```python
from build123d import *

# Parameters (mm, degrees)
SKETCH_1_W          = 9
SKETCH_1_H          = 6
EXTRUDE_1_DEPTH     = 1
SKETCH_2_W          = 1
SKETCH_2_H          = 2.206197562
EXTRUDE_2_DEPTH     = 12
CUT_EXTRUDE_1_DEPTH = 0.55
CUT_EXTRUDE_2_DEPTH = 0.55
CUT_EXTRUDE_3_DEPTH = 0.55
CUT_EXTRUDE_START   = -0.55
CUT_EXTRUDE_4_DEPTH = 0.55


with BuildPart() as part:
    # 草圖1 → 填料-伸長1 (new body)
    with BuildSketch(Plane(origin=(0, 0, 0), x_dir=(1, 0, 0), z_dir=(0, 1, 0))):
        Rectangle(SKETCH_1_W, SKETCH_1_H)
    extrude(amount=EXTRUDE_1_DEPTH)

    # 草圖2 → 填料-伸長2 (add)
    with BuildSketch(Plane(origin=(0, 1, 0), x_dir=(1, 0, 0), z_dir=(0, 1, 0))):
        with Locations((-4, 1.896901219)):
            Rectangle(SKETCH_2_W, SKETCH_2_H)
        with Locations((-4, -1.896901219)):
            Rectangle(SKETCH_2_W, SKETCH_2_H)
        with Locations((4, -1.896901219)):
            Rectangle(SKETCH_2_W, SKETCH_2_H)
        with Locations((4, 1.896901219)):
            Rectangle(SKETCH_2_W, SKETCH_2_H)
    extrude(amount=EXTRUDE_2_DEPTH)

    # 草圖4 → 除料-伸長1 (cut)
    with BuildSketch(Plane.XY.offset(-0.793802438)):
        with BuildLine():
            ThreePointArc((4.05, 11.897519797), (3.88890873, 12.286428527), (3.5, 12.447519797))
            Line((3.5, 12.447519797), (3.5, 11.897519797))
            Line((3.5, 11.897519797), (3.5, 11.347519797))
            ThreePointArc((3.5, 11.347519797), (3.88890873, 11.508611068), (4.05, 11.897519797))
        make_face()
        with BuildLine():
            Line((3.5, 11.897519797), (3.5, 12.447519797))
            ThreePointArc((3.5, 12.447519797), (2.95, 11.897519797), (3.5, 11.347519797))
            Line((3.5, 11.347519797), (3.5, 11.897519797))
        make_face()
    extrude(amount=-CUT_EXTRUDE_1_DEPTH, mode=Mode.SUBTRACT)

    # 草圖6 → 除料-伸長2 (cut)
    with BuildSketch(Plane(origin=(0, 0, 0.793802438), x_dir=(-1, 0, 0), z_dir=(0, 0, -1))):
        with BuildLine():
            ThreePointArc((-2.95, 11.9), (-3.11109127, 12.28890873), (-3.5, 12.45))
            Line((-3.5, 12.45), (-3.5, 11.9))
            Line((-3.5, 11.9), (-3.5, 11.35))
            ThreePointArc((-3.5, 11.35), (-3.11109127, 11.51109127), (-2.95, 11.9))
        make_face()
        with BuildLine():
            Line((-3.5, 11.9), (-3.5, 12.45))
            ThreePointArc((-3.5, 12.45), (-4.05, 11.9), (-3.5, 11.35))
            Line((-3.5, 11.35), (-3.5, 11.9))
        make_face()
    extrude(amount=-CUT_EXTRUDE_2_DEPTH, mode=Mode.SUBTRACT)

    # 草圖7 → 除料-伸長3 (cut)
    with BuildSketch(Plane(origin=(0, 0, 0.793802438), x_dir=(-1, 0, 0), z_dir=(0, 0, -1))):
        with BuildLine():
            ThreePointArc((4.05, 11.9), (3.88890873, 12.28890873), (3.5, 12.45))
            Line((3.5, 12.45), (3.5, 11.9))
            Line((3.5, 11.9), (3.5, 11.35))
            ThreePointArc((3.5, 11.35), (3.88890873, 11.51109127), (4.05, 11.9))
        make_face()
        with BuildLine():
            Line((3.5, 11.9), (3.5, 12.45))
            ThreePointArc((3.5, 12.45), (2.95, 11.9), (3.5, 11.35))
            Line((3.5, 11.35), (3.5, 11.9))
        make_face()
    extrude(amount=-CUT_EXTRUDE_3_DEPTH, mode=Mode.SUBTRACT)

    # 草圖8 → 除料-伸長4 (cut)
    with BuildSketch(Plane.XY.offset(-0.793802438).offset(CUT_EXTRUDE_START)):
        with BuildLine():
            ThreePointArc((-2.95, 11.9), (-3.11109127, 12.28890873), (-3.5, 12.45))
            Line((-3.5, 12.45), (-3.5, 11.9))
            Line((-3.5, 11.9), (-3.5, 11.35))
            ThreePointArc((-3.5, 11.35), (-3.11109127, 11.51109127), (-2.95, 11.9))
        make_face()
        with BuildLine():
            Line((-3.5, 11.9), (-3.5, 12.45))
            ThreePointArc((-3.5, 12.45), (-4.05, 11.9), (-3.5, 11.35))
            Line((-3.5, 11.35), (-3.5, 11.9))
        make_face()
    extrude(amount=CUT_EXTRUDE_4_DEPTH, mode=Mode.SUBTRACT)


solid = part.part
```
Design review of the part built by this model. Coordinates are the model's own, in mm. A direction names the side the tool comes from. Give positions to 0.01 mm unless a question says otherwise; leave off trailing zeros. Order: outer loops, then holes, each group sorted by start corner. A loop starts at its lowest first (then second) coordinate and runs counter-clockwise, first axis right, second up. Notation, with made-up numbers: (-1.5, 65) -> (25.5, 65) arc R24 cw to (25.5, 97) -> close; hole circle Ø1 at (9.5, 79). An arc over 180 degrees is marked (long way). Write each question's results on one line, items separated by ' | '. Start each with the question number.
Q1. Wall thickness on L1, parallel to X at y = 3, z = -1.05; L2, parallel to Z at x = 4, y = 11.5; L3, parallel to Y at x = -1, z = 0.5: over which ranges is each line inside the solid? List them lowest first. Write a range as from..to.
Q2. Mouldability with a two-part tool opening along X and no side actions: class faces 1 (the flat face through (3.5, 7, 2)), 2 (the flat face through (-3.5, 7, -2)), 3 (the flat face through (-4.5, 6, -1)), 4 (the flat face through (-4, 13, -2)) as +X half, -X half, draft (parallel to the pull), parting line (faces both ways), or undercut.
Q3. Add section C-C on x = 0. Give the boundary of the cut face in (y, z).
Q4. Add section A-A on y = 8.75. Give the boundary of the cut face in (x, z).
Q5. Machinability: for faces 5 (the flat face through (4, 7, -0.794)), 6 (the flat face through (0, 0, 0)), 7 (the flat face through (3.5, 7, -2)), which of the approach directions +Z, -Z, +X, -X, +Y, -Y give a long, thin tool a straight path to every point of the face, cutting with its end or side? Answer none if there is none.
Q6. For pin 1 (1.5 mm diameter, centred on x = 2.5, z = -2, fed in from -Y), flat-tipped, find the tip position at first contact; note if it passes through.
Q7. Add section B-B on z = 2. Give the boundary of the cut face in (x, y), and give its area (3 significant figures).
Q8. Add section D-D on z = 0.15. Give the boundary of the cut face in (x, y), and give its area (3 significant figures).
Found:
1) L1: x = -4.5..-3.5, 3.5..4.5 | L2: z = -3..-0.79, 0.79..3 | L3: y = 0..1
2) face 1: undercut | face 2: undercut | face 3: -X half | face 4: draft
3) outline: (0, -3) -> (1, -3) -> (1, 3) -> (0, 3) -> close
4) outline: (-4.5, -3) -> (-3.5, -3) -> (-3.5, -0.79) -> (-4.5, -0.79) -> close; (-4.5, 0.79) -> (-3.5, 0.79) -> (-3.5, 3) -> (-4.5, 3) -> close; (3.5, -3) -> (4.5, -3) -> (4.5, -0.79) -> (3.5, -0.79) -> close; (3.5, 0.79) -> (4.5, 0.79) -> (4.5, 3) -> (3.5, 3) -> close
5) face 5: +X, -X, +Y | face 6: +Z, -Z, +X, -X, -Y | face 7: +Z, -Z, +Y
6) pin 1: stops at y = 0
7) outline: (-4.5, 0) -> (4.5, 0) -> (4.5, 13) -> (3.5, 13) -> (3.5, 1) -> (-3.5, 1) -> (-3.5, 13) -> (-4.5, 13) -> close | area: 33.0 mm2
8) outline: (-4.5, 0) -> (4.5, 0) -> (4.5, 1) -> (-4.5, 1) -> close | area: 9.00 mm2
